Here's how the part is built. I have some questions about the finished solid (model axes, mm). A direction names the side the tool comes from. Round coordinates to 2 decimals unless told otherwise and drop trailing zeros. Write each loop counter-clockwise with the first axis right and the second up, starting at its lowest first coordinate (ties: lowest second). Pieces come first, ordered by that corner, then holes. Notation, with made-up numbers: (37, 52) - (83, 52) arc R19 ccw to (83, 88) - close; hole circle Ø7 at (5, 54). An arc over 180 degrees is marked (long way). Write item = value, one per line. Start each with the question number.
Item 1: If I drill on line 1 along Y through (x, z) = (-48, -10.5); line 2 along Z through (x, y) = (50, 104.5); line 3 along Z through (x, y) = (-49, 16), over which ranges is the centre line in solid material (lowest first)? Write a range as [from, to].
Item 2: For P1, Ø11, axis at y = 7, z = 33, coming from the +X side; P2, Ø1.5, axis at x = -46, z = -15, coming from the +Y side; P3, Ø11, axis at y = 5.5, z = 50, coming from the -X side, each with a flat end and sliding along its axis, tell me the tip position at first contact or that it passes through.
Item 3: If we section it at C-C (z = -60.5): Please give me the cut outline in (x, y).
Item 4: Which directions (+Z, -Z, +X, -X, +Y, -Y) give clear straight access to the entire face, cutting with the end or side of a thin tool? Please do faces 4 (the face through (-12.75, 5, 35)), 5 (the face through (2, 189, -60)), 6 (the face through (-50.428, 98.247, 31.356)).
Item 5: If we section it at B-B (y = 141.5): Please give me the cut outline in (x, z), and give its area (3 significant figures).
Item 6: If we section it at D-D (z = 43): Please give me the cut outline in (x, y).
Item 7: Thinking about a two-plate mould opening in X: for faces 1 (the face through (53.94, 98.25, 34.88)), 2 (the face through (3.3, 98.247, -64.195)), 3 (the face through (-15, 0, -2)), which applies, pulls with the +X half, pulls with the -X half, needs draft (parallel to the pull), parting line crosses it, or undercut?
Item 8: If we section it at A-A (z = 24): Please give me the cut outline in (x, y).
```python
from build123d import *

# Parameters (mm, degrees)
SKETCH_1_R          = 70
EXTRUDE_1_DEPTH     = 10
SKETCH_2_R          = 4
EXTRUDE_4_DEPTH     = 179
SKETCH_5_R          = 12.75
SKETCH_5_W          = 25.5
SKETCH_5_H          = 74.344778921
CUT_EXTRUDE_1_DEPTH = 10


with BuildPart() as part:
    # 草图1 → 凸台-拉伸1 (new body)
    with BuildSketch(Plane(origin=(0, 0, 0), x_dir=(1, 0, 0), z_dir=(0, 1, 0))):
        with Locations(Location((0, 0, 0), (0, 0, 270))):
            Circle(SKETCH_1_R)
    extrude(amount=EXTRUDE_1_DEPTH)

    # 草图2 → 凸台-拉伸4 (add)
    with BuildSketch(Plane(origin=(0, 10, 0), x_dir=(1, 0, 0), z_dir=(0, 1, 0))):
        with Locations(Location((-49.22649816, -35.171037501, 0), (0, 0, 90))):
            Circle(SKETCH_2_R)
        with Locations(Location((1.767528256, 60.5, 0), (0, 0, 90))):
            Circle(SKETCH_2_R)
        with Locations(Location((50.035340598, -34.010508542, 0), (0, 0, 90))):
            Circle(SKETCH_2_R)
    extrude(amount=EXTRUDE_4_DEPTH)

    # 草图5 → 切除-拉伸1 (cut)
    with BuildSketch(Plane(origin=(0, 10, 0), x_dir=(1, 0, 0), z_dir=(0, 1, 0))):
        Circle(SKETCH_5_R)
        with Locations((0, -37.17238946)):
            Rectangle(SKETCH_5_W, SKETCH_5_H)
    extrude(amount=-CUT_EXTRUDE_1_DEPTH, mode=Mode.SUBTRACT)


solid = part.part
```
Reply:
q1.line_1 = [0, 10]
q1.line_2 = [30.01, 38.01]
q1.line_3 = [31.18, 39.16]
q2.P1 = 64.37
q2.P2 = 10
q2.P3 = -54.03
q3.outline = (-35.21, 0) - (35.21, 0) - (35.21, 10) - (5.77, 10) - (5.77, 189) - (-2.23, 189) - (-2.23, 10) - (-35.21, 10) - close
q4.face_4 = +Z, +Y, -Y
q4.face_5 = +Z, -Z, +X, -X, +Y
q4.face_6 = +Y
q5.outline = circle Ø8 at (-49.23, 35.17); circle Ø8 at (1.77, -60.5); circle Ø8 at (50.04, 34.01)
q5.area = 151 mm2
q6.outline = (-55.24, 0) - (-12.75, 0) - (-12.75, 10) - (-55.24, 10) - close; (12.75, 0) - (55.24, 0) - (55.24, 10) - (12.75, 10) - close
q7.face_1 = undercut
q7.face_2 = parting line crosses it
q7.face_3 = needs draft
q8.outline = (-65.76, 0) - (-12.75, 0) - (-12.75, 10) - (-65.76, 10) - close; (12.75, 0) - (65.76, 0) - (65.76, 10) - (12.75, 10) - close
